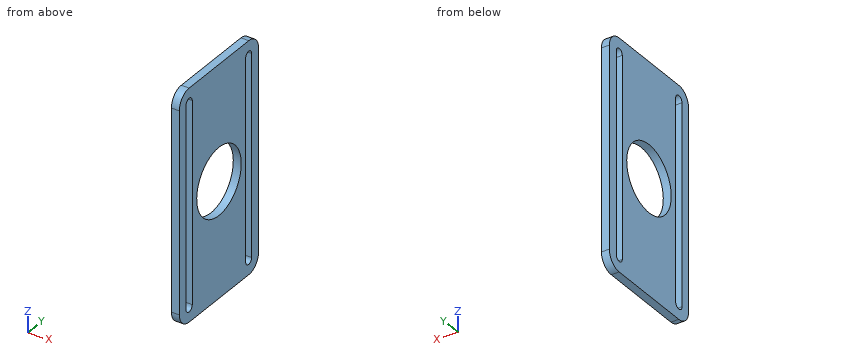
```python
from build123d import *

# Parameters (mm, degrees)
SKETCH_1_R      = 11.380487233
EXTRUDE_1_DEPTH = 2.7


with BuildPart() as part:
    # 草图1 → 凸台-拉伸1 (new body)
    with BuildSketch(Plane(origin=(0, 0, 0), x_dir=(0, 0, -1), z_dir=(1, 0, 0))):
        with BuildLine():
            Line((34, -5.005093632), (-34, -5.005093632))
            ThreePointArc((-34, -5.005093632), (-37.535533906, -3.540627537), (-39, -0.005093632))
            Line((-39, -0.005093632), (-39, 30.494906368))
            ThreePointArc((-39, 30.494906368), (-37.535533906, 34.030440274), (-34, 35.494906368))
            Line((-34, 35.494906368), (34, 35.494906368))
            ThreePointArc((34, 35.494906368), (37.535533906, 34.030440274), (39, 30.494906368))
            Line((39, 30.494906368), (39, -0.005093632))
            ThreePointArc((39, -0.005093632), (37.535533906, -3.540627537), (34, -5.005093632))
        make_face()
        with Locations(Location((0, 15.244906368, 0), (0, 0, 180))):
            Circle(SKETCH_1_R, mode=Mode.SUBTRACT)
        with BuildLine():
            Line((0, 1.594906368), (34, 1.594906368))
            ThreePointArc((34, 1.594906368), (35.6, -0.005093632), (34, -1.605093632))
            Line((34, -1.605093632), (0, -1.605093632))
            Line((0, -1.605093632), (-34, -1.605093632))
            ThreePointArc((-34, -1.605093632), (-35.6, -0.005093632), (-34, 1.594906368))
            Line((-34, 1.594906368), (0, 1.594906368))
        make_face(mode=Mode.SUBTRACT)
        with BuildLine():
            Line((0, 31.922276961), (34, 31.922276961))
            ThreePointArc((34, 31.922276961), (35.513685296, 30.408591665), (34, 28.894906368))
            Line((34, 28.894906368), (0, 28.894906368))
            Line((0, 28.894906368), (-34, 28.894906368))
            ThreePointArc((-34, 28.894906368), (-35.513685296, 30.408591665), (-34, 31.922276961))
            Line((-34, 31.922276961), (0, 31.922276961))
        make_face(mode=Mode.SUBTRACT)
    extrude(amount=EXTRUDE_1_DEPTH)


solid = part.part
```
Build history of the part. All positions in model axes, mm. Round coordinates to 2 decimals unless told otherwise and drop trailing zeros. Order: outer loops, then holes, each group sorted by start corner. A loop starts at its lowest first (then second) coordinate and runs counter-clockwise, first axis right, second up. Notation, with made-up numbers: (65, 5) - (104, 5) arc R13 cw to (104, 15) - close; hole circle Ø5 at (-7, 44.25). An arc over 180 degrees is marked (long way). Use a Markdown table: item, result.
1) Saw through at C-C on z = -16.5. Write the cut outline in (x, y).
Recorded:
| item | result |
|---|---|
| outline | (0, -5.01) - (2.7, -5.01) - (2.7, -1.61) - (0, -1.61) - close; (0, 1.59) - (2.7, 1.59) - (2.7, 28.89) - (0, 28.89) - close; (0, 31.92) - (2.7, 31.92) - (2.7, 35.49) - (0, 35.49) - close |
2) Saw through at D-D on x = 0.5. Write the cut outline in (y, z).
Recorded:
| item | result |
|---|---|
| outline | (-5.01, -34) arc R5 ccw to (-0.01, -39) - (30.49, -39) arc R5 ccw to (35.49, -34) - (35.49, 34) arc R5 ccw to (30.49, 39) - (-0.01, 39) arc R5 ccw to (-5.01, 34) - close; hole (-1.61, -34) arc R1.6 ccw to (1.59, -34) - (1.59, 34) arc R1.6 ccw to (-1.61, 34) - close; hole circle Ø22.76 at (15.24, 0); hole (28.89, -34) arc R1.51 ccw to (31.92, -34) - (31.92, 34) arc R1.51 ccw to (28.89, 34) - close |
3) Wall check: L1, parallel to Y at x = 1.25, z = 0; L2, parallel to Y at x = 2, z = 29.5; L3, parallel to Z at x = 2.05, y = 21.5. Give the ranges that are in metal, low to high.
Recorded:
| item | result |
|---|---|
| L1 | y = -5.01 to -1.61, 1.59 to 3.86, 26.63 to 28.89, 31.92 to 35.49 |
| L2 | y = -5.01 to -1.61, 1.59 to 28.89, 31.92 to 35.49 |
| L3 | z = -39 to -9.51, 9.51 to 39 |
4) Saw through at A-A on z = 0. Write the cut outline in (x, y), and give its area (3 significant figures).
Recorded:
| item | result |
|---|---|
| outline | (0, -5.01) - (2.7, -5.01) - (2.7, -1.61) - (0, -1.61) - close; (0, 1.59) - (2.7, 1.59) - (2.7, 3.86) - (0, 3.86) - close; (0, 26.63) - (2.7, 26.63) - (2.7, 28.89) - (0, 28.89) - close; (0, 31.92) - (2.7, 31.92) - (2.7, 35.49) - (0, 35.49) - close |
| area | 31.1 mm² |
5) Saw through at B-B on y = 6.5. Write the cut outline in (x, z).
Recorded:
| item | result |
|---|---|
| outline | (0, -39) - (2.7, -39) - (2.7, -7.28) - (0, -7.28) - close; (0, 7.28) - (2.7, 7.28) - (2.7, 39) - (0, 39) - close |
